Build history of the part. All positions in model axes, mm. Give positions to 0.01 mm unless a question says otherwise; leave off trailing zeros. Order: outer loops, then holes, each group sorted by start corner. A loop starts at its lowest first (then second) coordinate and runs counter-clockwise, first axis right, second up. Notation, with made-up numbers: (85.25, 30.5) - (109.25, 30.5) arc R17 cw to (109.25, 48.5) - close; hole circle Ø2 at (-36, 75). An arc over 180 degrees is marked (long way). Use a Markdown table: item, result.
from build123d import *

# Parameters (mm, degrees)
CROQUIS1_R              = 1.498200291
CROQUIS1_R_2            = 1.5
SALIENTE_EXTRUIR1_DEPTH = 1.5


with BuildPart() as part:
    # Croquis1 → Saliente-Extruir1 (new, symmetric)
    with BuildSketch(Plane(origin=(0, 0, 0), x_dir=(1, 0, 0), z_dir=(0, 1, 0))):
        with BuildLine():
            Line((-7.044335514, 8.976515941), (12.614040425, 8.976515941))
            ThreePointArc((12.614040425, 8.976515941), (14.381807378, 8.244282894), (15.114040425, 6.476515941))
            Line((15.114040425, 6.476515941), (15.114040425, -15.544827048))
            ThreePointArc((15.114040425, -15.544827048), (14.381807378, -17.312594001), (12.614040425, -18.044827048))
            Line((12.614040425, -18.044827048), (-7.044335514, -18.044827048))
            ThreePointArc((-7.044335514, -18.044827048), (-8.812102467, -17.312594001), (-9.544335514, -15.544827048))
            Line((-9.544335514, -15.544827048), (-9.544335514, 6.476515941))
            ThreePointArc((-9.544335514, 6.476515941), (-8.812102467, 8.244282894), (-7.044335514, 8.976515941))
        make_face()
        with Locations(Location((2.784852456, 6.465844447, 0), (0, 0, 270))):
            Circle(CROQUIS1_R, mode=Mode.SUBTRACT)
        with Locations(Location((2.784852456, -15.534155553, 0), (0, 0, 90))):
            Circle(CROQUIS1_R, mode=Mode.SUBTRACT)
        with Locations(Location((-6.290312273, 6.400402587, 0), (0, 0, 270))):
            Circle(CROQUIS1_R_2, mode=Mode.SUBTRACT)
        with Locations(Location((-6.290312273, -15.468713694, 0), (0, 0, 90))):
            Circle(CROQUIS1_R_2, mode=Mode.SUBTRACT)
        with Locations(Location((11.860017184, -15.468713694, 0), (0, 0, 270))):
            Circle(CROQUIS1_R_2, mode=Mode.SUBTRACT)
        with Locations(Location((11.860017184, 6.400402587, 0), (0, 0, 90))):
            Circle(CROQUIS1_R_2, mode=Mode.SUBTRACT)
    extrude(amount=SALIENTE_EXTRUIR1_DEPTH, both=True)


solid = part.part
1) Two-plate mould, pull along X, no slides. Class faces 1 (the cylindrical face through (-5.38, -0.02, 16.66)), 2 (the flat face through (3, 0, -8.977)), 3 (the cylindrical face through (-8.831, 0.021, -8.225)), 4 (the flat face through (15.114, 0, 4)): +X half, -X half, draft (parallel to the pull), parting line (faces both ways), or undercut.
Computed:
| item | result |
|---|---|
| face 1 | undercut |
| face 2 | draft |
| face 3 | -X half |
| face 4 | +X half |
2) Pin check, flat tip, straight feed: P1, Ø2.5, axis at x = -6.29, z = 15.47, coming from the -Y side. Stop position of the tip, or through.
Computed:
| item | result |
|---|---|
| P1 | passes through |
3) Wall check: line 1 (X direction, y = -0.1, z = -5.25); line 2 (Z direction, x = 12.75, y = -0.5); line 3 (Z direction, x = 12.25, y = -0.3). Give the ranges that are in metal, low to high. Write a range as from..to.
Computed:
| item | result |
|---|---|
| line 1 | x = -9.54..-7.25, -5.33..1.91, 3.66..10.9, 12.82..15.11 |
| line 2 | z = -8.97..-7.61, -5.19..14.26, 16.68..18.04 |
| line 3 | z = -8.98..-7.85, -4.95..14.02, 16.92..18.04 |
4) Slice it at A-A (y = -0.35). Write the cut outline in (x, z), and give its area (3 significant figures).
Computed:
| item | result |
|---|---|
| outline | (-9.54, -6.48) arc R2.5 ccw to (-7.04, -8.98) - (12.61, -8.98) arc R2.5 ccw to (15.11, -6.48) - (15.11, 15.54) arc R2.5 ccw to (12.61, 18.04) - (-7.04, 18.04) arc R2.5 ccw to (-9.54, 15.54) - close; hole circle Ø3 at (-6.29, -6.4); hole circle Ø3 at (-6.29, 15.47); hole circle Ø3 at (2.78, -6.47); hole circle Ø3 at (2.78, 15.53); hole circle Ø3 at (11.86, -6.4); hole circle Ø3 at (11.86, 15.47) |
| area | 619 mm² |
5) Slice it at B-B (x = 11.25). Write the cut outline in (y, z).
Computed:
| item | result |
|---|---|
| outline | (-1.5, -8.98) - (1.5, -8.98) - (1.5, -7.77) - (-1.5, -7.77) - close; (-1.5, -5.03) - (1.5, -5.03) - (1.5, 14.1) - (-1.5, 14.1) - close; (-1.5, 16.84) - (1.5, 16.84) - (1.5, 18.04) - (-1.5, 18.04) - close |
